from build123d import *

# Parameters (mm, degrees)
SKETCH1_W               = 152.4
SKETCH1_H               = 171.45
BOSS_EXTRUDE1_DEPTH     = 12.7
CUT_EXTRUDE1_DEPTH      = 230.743666942
CUT_EXTRUDE1_DEPTH_BACK = 230.743666942
SKETCH2_R               = 26.67
CUT_EXTRUDE2_DEPTH      = 230.743666942
CUT_EXTRUDE2_DEPTH_BACK = 230.743666942
SKETCH3_R               = 3.175
SKETCH4_R               = 29.401540703
CUT_EXTRUDE3_DEPTH      = 2.54
CUT_EXTRUDE4_DEPTH      = 230.743666942
CUT_EXTRUDE4_DEPTH_BACK = 230.743666942
SKETCH5_W               = 76.2
SKETCH5_H               = 88.9
CUT_EXTRUDE5_DEPTH      = 230.743666942
CUT_EXTRUDE5_DEPTH_BACK = 230.743666942
SKETCH7_R               = 3.175


with BuildPart() as part:
    # Sketch1 → Boss-Extrude1 (new body)
    with BuildSketch(Plane(origin=(0, 0, 0), x_dir=(1, 0, 0), z_dir=(0, 1, 0))):
        with Locations((-76.2, 85.725)):
            Rectangle(SKETCH1_W, SKETCH1_H)
    extrude(amount=BOSS_EXTRUDE1_DEPTH)

    # Sketch2 → Cut-Extrude1 (cut, two sides: drawn at the far end of the back side and taken through both)
    with BuildSketch(Plane(origin=(0, 12.7, 0), x_dir=(1, 0, 0), z_dir=(0, 1, 0)).offset(-CUT_EXTRUDE1_DEPTH_BACK)):
        with Locations(Location((-76.2, 133.35, 0), (0, 0, 270))):
            Circle(SKETCH2_R)
    extrude(amount=CUT_EXTRUDE1_DEPTH + CUT_EXTRUDE1_DEPTH_BACK, mode=Mode.SUBTRACT)

    # Sketch3 → Cut-Extrude2 (cut, two sides: drawn at the far end of the back side and taken through both)
    with BuildSketch(Plane(origin=(0, 12.7, 0), x_dir=(1, 0, 0), z_dir=(0, 1, 0)).offset(-CUT_EXTRUDE2_DEPTH_BACK)):
        with Locations(Location((-139.7, 158.75, 0), (0, 0, 270))):
            Circle(SKETCH3_R)
        with Locations(Location((-12.7, 158.75, 0), (0, 0, 270))):
            Circle(SKETCH3_R)
        with Locations(Location((-12.7, 95.25, 0), (0, 0, 270))):
            Circle(SKETCH3_R)
        with Locations(Location((-139.7, 95.25, 0), (0, 0, 270))):
            Circle(SKETCH3_R)
    extrude(amount=CUT_EXTRUDE2_DEPTH + CUT_EXTRUDE2_DEPTH_BACK, mode=Mode.SUBTRACT)

    # Sketch4 → Cut-Extrude3 (cut)
    with BuildSketch(Plane(origin=(0, 12.7, 0), x_dir=(1, 0, 0), z_dir=(0, 1, 0))):
        with Locations(Location((-76.2, 133.35, 0), (0, 0, 270))):
            Circle(SKETCH4_R)
    extrude(amount=-CUT_EXTRUDE3_DEPTH, mode=Mode.SUBTRACT)

    # Sketch5 → Cut-Extrude4 (cut, two sides: drawn at the far end of the back side and taken through both)
    with BuildSketch(Plane.XZ.offset(-CUT_EXTRUDE4_DEPTH_BACK)):
        with Locations((-76.2, -44.45)):
            Rectangle(SKETCH5_W, SKETCH5_H)
    extrude(amount=CUT_EXTRUDE4_DEPTH + CUT_EXTRUDE4_DEPTH_BACK, mode=Mode.SUBTRACT)

    # Sketch7 → Cut-Extrude5 (cut, two sides: drawn at the far end of the back side and taken through both)
    with BuildSketch(Plane.XZ.offset(-CUT_EXTRUDE5_DEPTH_BACK)):
        with Locations(Location((-19.05, -12.7, 0), (0, 0, 270))):
            Circle(SKETCH7_R)
        with Locations(Location((-133.35, -12.7, 0), (0, 0, 270))):
            Circle(SKETCH7_R)
    extrude(amount=CUT_EXTRUDE5_DEPTH + CUT_EXTRUDE5_DEPTH_BACK, mode=Mode.SUBTRACT)


solid = part.part
Work out the finished part from the listing and answer in its coordinate system (mm). A direction names the side the tool comes from. Coordinates: 2 decimals unless noted, no trailing zeros. Write each loop counter-clockwise with the first axis right and the second up, starting at its lowest first coordinate (ties: lowest second). Pieces come first, ordered by that corner, then holes.
1. Consider line 1 along X through (y, z) = (6.75, -12.7) (3 decimals); line 2 along Z through (x, y) = (-139.7, 8.75) (3 decimals); line 3 along X through (y, z) = (7, -95.25) (3 decimals). Determine where each line is inside the solid, lowest interval first.
Results list:
line 1: x = -152.4 to -136.525, -130.175 to -114.3, -38.1 to -22.225, -15.875 to 0
line 2: z = -171.45 to -161.925, -155.575 to -98.425, -92.075 to 0
line 3: x = -152.4 to -142.875, -136.525 to -15.875, -9.525 to 0
2. The part is cut by section C-C, the plane y = 4.75. Write down the section's boundary in (x, z) (3 decimals), and give its area (3 significant figures).
Results list:
outline: (-152.4, -171.45) - (0, -171.45) - (0, 0) - (-38.1, 0) - (-38.1, -88.9) - (-114.3, -88.9) - (-114.3, 0) - (-152.4, 0) - close; hole circle Ø6.35 at (-139.7, -158.75); hole circle Ø6.35 at (-139.7, -95.25); hole circle Ø6.35 at (-133.35, -12.7); hole circle Ø53.34 at (-76.2, -133.35); hole circle Ø6.35 at (-19.05, -12.7); hole circle Ø6.35 at (-12.7, -158.75); hole circle Ø6.35 at (-12.7, -95.25)
area: 16,900 mm2
3. Flat-ended cylindrical pins translate along their axes: pin 1 (5 mm diameter, centred on x = -139.7, z = -95.25, fed in from -Y); pin 2 (6.5 mm diameter, centred on x = -62.5, y = 8, fed in from +Z). Find the tip coordinate at first contact, or state that the pin passes through.
Results list:
pin 1: passes through
pin 2: stops at z = -88.9
4. For a pull along Z with two mould halves and no side action, classify faces 1 (the flat face through (-38.1, 6, -45)), 2 (the cylindrical face through (-94.09, 11.45, -156.68)), 3 (the flat face through (-134, 6, 0)) as +Z half, -Z half, draft (parallel to the pull), parting line (faces both ways), or undercut.
Results list:
face 1: draft
face 2: undercut
face 3: +Z half
5. The part is cut by section A-A, the plane x = -19.05. Write down the section's boundary in (y, z) (3 decimals), and give its area (3 significant figures).
Results list:
outline: (0, -171.45) - (12.7, -171.45) - (12.7, -15.875) - (0, -15.875) - close; (0, -9.525) - (12.7, -9.525) - (12.7, 0) - (0, 0) - close
area: 2,100 mm2
6. The part is cut by section D-D, the plane z = -95.25. Write down the section's boundary in (x, y) (3 decimals), and give its area (3 significant figures).
Results list:
outline: (-152.4, 0) - (-142.875, 0) - (-142.875, 12.7) - (-152.4, 12.7) - close; (-136.525, 0) - (-15.875, 0) - (-15.875, 12.7) - (-136.525, 12.7) - close; (-9.525, 0) - (0, 0) - (0, 12.7) - (-9.525, 12.7) - close
area: 1,770 mm2
7. For faces 4 (the cylindrical face through (-75.027, 5.009, -159.994)), 5 (the flat face through (-102.2, 10.16, -140)), 6 (the flat face through (-114.3, 6, -45)), determine the directions among +Z, -Z, +X, -X, +Y, -Y from which every point of the face is accessible in a straight line to the end or side of a thin tool.
Results list:
face 4: +Y, -Y
face 5: +Y
face 6: +Z, +Y, -Y
8. The part is cut by section B-B, the plane z = -133.35. Write down the section's boundary in (x, y).
Results list:
outline: (-152.4, 0) - (-102.87, 0) - (-102.87, 10.16) - (-105.6, 10.16) - (-105.6, 12.7) - (-152.4, 12.7) - close; (-49.53, 0) - (0, 0) - (0, 12.7) - (-46.8, 12.7) - (-46.8, 10.16) - (-49.53, 10.16) - close
